Work out the finished part from the listing and answer in its coordinate system (mm). Round coordinates to 2 decimals unless told otherwise and drop trailing zeros. Order: outer loops, then holes, each group sorted by start corner. A loop starts at its lowest first (then second) coordinate and runs counter-clockwise, first axis right, second up.
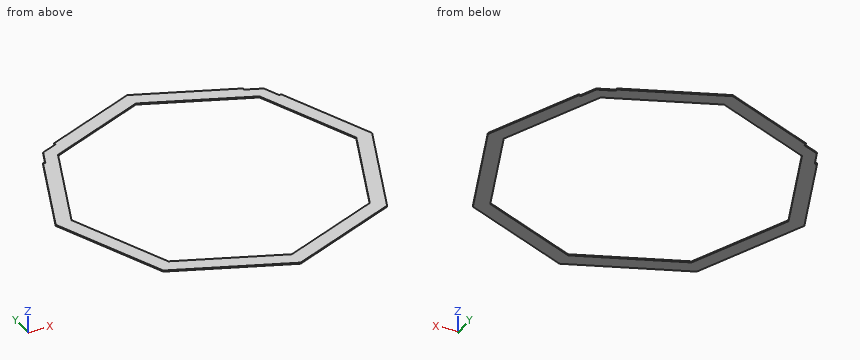
Autodesk Inventor part; units mm, degrees
ref_plane "YZ Plane" through (0, 0, 0) normal (1, 0, 0) x (0, 1, 0)
ref_plane "XZ Plane" through (0, 0, 0) normal (0, 1, 0) x (-1, 0, 0)
ref_plane "XY Plane" through (0, 0, 0) normal (0, 0, 1) x (1, 0, 0)
sketch "Sketch1" plane through (0, 0, 0) normal (0, 0, 1) x (1, 0, 0)
  line L0 (1.1481, 270.1225) -> (190.1937, 191.8173)
  line L1 (191.8173, 190.1937) -> (270.1225, 1.1481)
  line L2 (270.1225, -1.1481) -> (191.8173, -190.1937)
  line L3 (190.1937, -191.8173) -> (1.1481, -270.1225)
  line L4 (-1.1481, -270.1225) -> (-190.1937, -191.8173)
  line L5 (-191.8173, -190.1937) -> (-270.1225, -1.1481)
  line L6 (-270.1225, 1.1481) -> (-191.8173, 190.1937)
  line L7 (-190.1937, 191.8173) -> (-1.1481, 270.1225)
  line L8 (172.2075, 172.2075) -> (0, 243.5382)
  line L9 (0, 243.5382) -> (-172.2075, 172.2075)
  line L10 (-172.2075, 172.2075) -> (-243.5382, 0)
  line L11 (-243.5382, 0) -> (-172.2075, -172.2075)
  line L12 (-172.2075, -172.2075) -> (0, -243.5382)
  line L13 (0, -243.5382) -> (172.2075, -172.2075)
  line L14 (172.2075, -172.2075) -> (243.5382, 0)
  line L15 (243.5382, 0) -> (172.2075, 172.2075)
  arc A0 (1.1481, 270.1225) -> (-1.1481, 270.1225) centre (0, 267.3509) ccw
  arc A1 (-190.1937, 191.8173) -> (-191.8173, 190.1937) centre (-189.0456, 189.0456) ccw
  arc A2 (-270.1225, 1.1481) -> (-270.1225, -1.1481) centre (-267.3509, 0) ccw
  arc A3 (-191.8173, -190.1937) -> (-190.1937, -191.8173) centre (-189.0456, -189.0456) ccw
  arc A4 (-1.1481, -270.1225) -> (1.1481, -270.1225) centre (0, -267.3509) ccw
  arc A5 (190.1937, -191.8173) -> (191.8173, -190.1937) centre (189.0456, -189.0456) ccw
  arc A6 (270.1225, -1.1481) -> (270.1225, 1.1481) centre (267.3509, 0) ccw
  arc A7 (191.8173, 190.1937) -> (190.1937, 191.8173) centre (189.0456, 189.0456) ccw
  point P0 (0, 0)
  point P1 (0, 0)
  point P2 (0, 270.5981)
  point P3 (191.3417, 191.3417)
  point P4 (270.5981, 0)
  point P5 (191.3417, -191.3417)
  point P6 (0, -270.5981)
  point P7 (-191.3417, -191.3417)
  point P8 (-270.5981, 0)
  point P9 (-191.3417, 191.3417)
  dimension "d18" = 500
  dimension "d19" = 25
  dimension "d20" = 3
  dimension "d22" = 3
extrude "Plate2" add sketch "Sketch1" against normal blind 2
sketch "Sketch3" plane through (0, 0, 0) normal (0, 0, 1) x (1, 0, 0)
  line L0 (-191.8173, 190.1937) -> (-270.1225, 1.1481)
  arc A0 (-190.1937, 191.8173) -> (-191.8173, 190.1937) centre (-189.0456, 189.0456) ccw
  line L1 (-1.1481, 270.1225) -> (-190.1937, 191.8173)
  line L2 (-200.2363, 160.7224) -> (-189.1385, 187.5149)
  line L3 (-187.5149, 189.1385) -> (-160.7224, 200.2363)
  arc A1 (-187.5149, 189.1385) -> (-189.1385, 187.5149) centre (-186.3668, 186.3668) ccw
  line L4 (-162.0618, 203.4699) -> (-160.7224, 200.2363)
  line L5 (-200.2363, 160.7224) -> (-203.4699, 162.0618)
  point P0 (0, 0)
  dimension "d23" = 3.5
  dimension "d24" = 3
  dimension "d25" = 29
  dimension "d26" = 3.5
extrude "Extrusion1" cut sketch "Sketch3" against normal up to surface (2 mm away)
mirror "Mirror1" about plane through (0, 0, 0) normal (1, 0, 0) of "Extrusion1"
equation "\"d22\" = d20"
equation "\"d21\" = Thickness"
equation "\"BendRadius\" = Thickness"
equation "\"BendReliefWidth\" = Thickness"
equation "\"BendReliefDepth\" = 0.5 * Thickness"
equation "\"CornerReliefSize\" = 4 * Thickness"
equation "\"MinimumRemnant\" = 2 * Thickness"
equation "\"TransitionRadius\" = BendRadius"
equation "\"JacobiRadiusSize\" = BendRadius"
equation "\"GapSize\" = Thickness"
properties part number "ДМС 104.1 Сектор кольца усилителя барабана полный"
Item 1: Find section C-C (y = -209.5). Write down the section's boundary in (x, z), plus the area to 3 significant figures.
Item 2: Find section A-A (x = -222). Write down the section's boundary in (y, z), plus the area to 3 significant figures.
Item 3: Find the intervals of material crossed by line 1 along Y through (x, z) = (-0.5, -1.6); line 2 along Y through (x, z) = (-229, -1.4), in increasing order.
Model answer:
1. outline: (-147.5, -2) - (-82.18, -2) - (-82.18, 0) - (-147.5, 0) - close; (82.18, -2) - (147.5, -2) - (147.5, 0) - (82.18, 0) - close
1. area: 261 mm2
2. outline: (-117.33, -2) - (-52, -2) - (-52, 0) - (-117.33, 0) - close; (52, -2) - (117.33, -2) - (117.33, 0) - (52, 0) - close
2. area: 261 mm2
3. line 1: y = -270.31 to -243.33, 243.33 to 270.31
3. line 2: y = -100.43 to -35.1, 35.1 to 100.43
